```python
from build123d import *

# Parameters (mm, degrees)
SKETCH_1_R          = 15
SKETCH_1_R_2        = 4.1
EXTRUDE_1_DEPTH     = 4
SKETCH_2_R          = 7
SKETCH_2_R_2        = 4.1
EXTRUDE_2_DEPTH     = 17
SKETCH_5_R          = 2
CUT_EXTRUDE_1_DEPTH = 12
SKETCH_7_R          = 1.5
CUT_EXTRUDE_3_DEPTH = 4
CHAMFER_1_SIZE      = 1


with BuildPart() as part:
    # Sketch 1 → Extrude 1 (new body)
    with BuildSketch(Plane(origin=(0, 0, 0), x_dir=(1, 0, 0), z_dir=(0, 1, 0))):
        with Locations(Location((0, 0, 0), (0, 0, 270))):
            Circle(SKETCH_1_R)
        with Locations(Location((0, 0, 0), (0, 0, 270))):
            Circle(SKETCH_1_R_2, mode=Mode.SUBTRACT)
    extrude(amount=EXTRUDE_1_DEPTH)

    # Sketch 2 → Extrude 2 (add)
    with BuildSketch(Plane(origin=(0, 4, 0), x_dir=(1, 0, 0), z_dir=(0, 1, 0))):
        with Locations(Location((0, 0, 0), (0, 0, 270))):
            Circle(SKETCH_2_R)
        with Locations(Location((0, 0, 0), (0, 0, 270))):
            Circle(SKETCH_2_R_2, mode=Mode.SUBTRACT)
    extrude(amount=EXTRUDE_2_DEPTH)

    # Sketch 5 → Cut-Extrude 1 (cut)
    with BuildSketch(Plane.ZY):
        with Locations((0, 7.5)):
            Circle(SKETCH_5_R)
    extrude(amount=-CUT_EXTRUDE_1_DEPTH, mode=Mode.SUBTRACT)

    # Sketch 7 → Cut-Extrude 3 (cut)
    with BuildSketch(Plane(origin=(0, 4, 0), x_dir=(1, 0, 0), z_dir=(0, 1, 0))):
        with Locations(Location((12, 0, 0), (0, 0, 270))):
            Circle(SKETCH_7_R)
        with Locations(Location((0, -12, 0), (0, 0, 270))):
            Circle(SKETCH_7_R)
        with Locations(Location((-12, 0, 0), (0, 0, 270))):
            Circle(SKETCH_7_R)
        with Locations(Location((0, 12, 0), (0, 0, 270))):
            Circle(SKETCH_7_R)
    extrude(amount=-CUT_EXTRUDE_3_DEPTH, mode=Mode.SUBTRACT)

    # Chamfer 1
    chamfer_1_edges = [part.edges().sort_by_distance(p)[0] for p in [
        (0, 21, -4.1),
    ]]
    chamfer(chamfer_1_edges, length=CHAMFER_1_SIZE)


solid = part.part
```
Part model, mm, in its own coordinate system. A direction names the side the tool comes from. Give positions to 0.01 mm unless a question says otherwise; leave off trailing zeros. Order: outer loops, then holes, each group sorted by start corner. A loop starts at its lowest first (then second) coordinate and runs counter-clockwise, first axis right, second up. Notation, with made-up numbers: (-6, 83.25) - (0, 83.25) arc R29 ccw to (0, 120.25) - close; hole circle Ø1 at (78.5, -37). An arc over 180 degrees is marked (long way). Use one line per item in the form item = value.
Item 1: Two-plate mould, pull along X, no slides. Class faces 1 (the face through (0.07, 2.03, -13.5)), 2 (the face through (-3.1, 4, 6.5)), 3 (the face through (-6.21, 12.38, 3.23)): released by +X, released by -X, zero draft, split by the parting line, or undercut.
Solution:
face_1 = undercut
face_2 = zero draft
face_3 = split by the parting line
Item 2: Slice it at D-D on z = -12.5. Give the cut face in (x, y).
Solution:
outline = (-8.29, 0) - (-1.41, 0) - (-1.41, 4) - (-8.29, 4) - close; (1.41, 0) - (8.29, 0) - (8.29, 4) - (1.41, 4) - close
Item 3: Which spindle directions (+Z, -Z, +X, -X, +Y, -Y) get a long thin tool onto all of the face, cutting with end or side? Do faces 4 (the face through (0.07, 2.03, 10.5)), 5 (the face through (5.27, 9.483, -0.26)). Say none if no direction does.
Solution:
face_4 = +Y, -Y
face_5 = +X
Item 4: Slice it at A-A on z = 0. Give the cut face in (x, y), and give its area (3 significant figures).
Solution:
outline = (-15, 0) - (-13.5, 0) - (-13.5, 4) - (-15, 4) - close; (-10.5, 0) - (-4.1, 0) - (-4.1, 20) - (-5.1, 21) - (-7, 21) - (-7, 4) - (-10.5, 4) - close; (4.1, 0) - (10.5, 0) - (10.5, 4) - (7, 4) - (7, 5.5) - (4.1, 5.5) - close; (4.1, 9.5) - (7, 9.5) - (7, 21) - (5.1, 21) - (4.1, 20) - close; (13.5, 0) - (15, 0) - (15, 4) - (13.5, 4) - close
area = 149 mm2
Item 5: Pin check, flat tips, straight feed: pin 1 Ø10 at (x, y) = (2.5, 9.5) entering from -Z; pin 2 Ø8 at (x, y) = (-7, 18) entering from -Z; pin 3 Ø1.5 at (x, z) = (4.5, -9.5) entering from +Y; pin 4 Ø2.5 at (x, z) = (0, -12) entering from -Y. Stop position of each tip, or through.
Solution:
pin_1 = -7
pin_2 = -6.32
pin_3 = 4
pin_4 = through
Item 6: Slice it at C-C on x = 0. Give the cut face in (y, z), and give its area (3 significant figures).
Solution:
outline = (0, -15) - (4, -15) - (4, -13.5) - (0, -13.5) - close; (0, -10.5) - (4, -10.5) - (4, -7) - (21, -7) - (21, -5.1) - (20, -4.1) - (0, -4.1) - close; (0, 4.1) - (20, 4.1) - (21, 5.1) - (21, 7) - (4, 7) - (4, 10.5) - (0, 10.5) - close; (0, 13.5) - (4, 13.5) - (4, 15) - (0, 15) - close
area = 161 mm2
Item 7: Slice it at B-B on x = -12. Give the cut face in (y, z), and give its area (3 significant figures).
Solution:
outline = (0, -9) - (4, -9) - (4, -1.5) - (0, -1.5) - close; (0, 1.5) - (4, 1.5) - (4, 9) - (0, 9) - close
area = 60.0 mm2
Item 8: Probe probe 1 along X at (y, z) = (18.5, 0.25); probe 2 along Y at (x, z) = (-10, 5.5); probe 3 along Z at (x, y) = (6, 7.5). List the from-to ranges inside material, lowest first. Write a range as from..to.
Solution:
probe_1 = -7..-4.09, 4.09..7
probe_2 = 0..4
probe_3 = -3.61..-2, 2..3.61
